Autodesk Inventor part; units mm, degrees
ref_plane "YZ Plane" through (0, 0, 0) normal (1, 0, 0) x (0, 1, 0)
ref_plane "XZ Plane" through (0, 0, 0) normal (0, 1, 0) x (-1, 0, 0)
ref_plane "XY Plane" through (0, 0, 0) normal (0, 0, 1) x (1, 0, 0)
sketch "Sketch1" plane through (0, 0, 0) normal (0, 0, 1) x (1, 0, 0)
  circle A0 centre (0, 0) radius 25
  circle A1 centre (0, 0) radius 35
  line L0 (-17.6777, 17.6777) -> (-24.7487, 24.7487)
  line L1 (0, 35) -> (0, 0) construction
  line L2 (-24.0315, 25.4457) -> (-16.9564, 18.3706)
  line L3 (-1.1667, 34.9806) -> (-1.1667, 34.9972)
  line L4 (1.1667, 34.9806) -> (1.1667, 34.9972)
  line L5 (17.6777, 17.6777) -> (24.7487, 24.7487)
  line L6 (24.0315, 25.4457) -> (16.9564, 18.3706)
  line L7 (-25.4457, 24.0315) -> (-18.3706, 16.9564)
  line L8 (25.4457, 24.0315) -> (18.3706, 16.9564)
  line L9 (-1, 15) -> (1, 15)
  line L10 (1, 15) -> (1, 0)
  line L11 (1, 0) -> (-1, 0)
  line L12 (-1, 0) -> (-1, 15)
  line L13 (-1, 0) -> (1, 0)
  line L14 (1, 0) -> (1, -6)
  line L15 (1, -6) -> (-1, -6)
  line L16 (-1, -6) -> (-1, 0)
  line L17 (-1, -6) -> (-5, -6)
  line L18 (-5, -6) -> (-5, 3)
  line L19 (-5, 3) -> (-1, 3)
  line L20 (-1, 3) -> (-1, -6)
  line L21 (-5, 3) -> (-21.2192, -13.2192)
  line L22 (-5, -6) -> (-17.1706, -18.1706)
  line L23 (-5, 3) -> (-1, 15)
  line L24 (-5, -6) -> (-1, -2)
  line L25 (1, 0) -> (1, 15)
  line L26 (1, -6) -> (1, 0)
  line L27 (5, 3) -> (21.2192, -13.2192)
  line L28 (5, -6) -> (17.1706, -18.1706)
  line L29 (5, 3) -> (1, 15)
  line L30 (5, -6) -> (1, -2)
  point P0 (-20.5061, 21.9203)
  point P1 (-21.9203, 20.5061)
  point P2 (20.5061, 21.9203)
  point P3 (21.9203, 20.5061)
  point P4 (-1, -2)
  point P5 (1, 0)
  point P6 (1, -2)
  dimension "d0" = 50
  dimension "d1" = 10
  dimension "d2" = 45
  dimension "d3" = 1
  dimension "d5" = 2
  dimension "d6" = 15
  dimension "d7" = 6
  dimension "d8" = 2
  dimension "d9" = 4
  dimension "d11" = 45
  dimension "d12" = 45
  dimension "d13" = 3
  dimension "d14" = 45
extrude "Extrusion1" add sketch "Sketch1" along normal blind 5 contours A0 L0 A1 L2 | A1 L0 A0 L7
sketch "Sketch3" plane through (-24.0315, 25.4457, 0) normal (0.7071, 0.7071, 0) x (-0.7071, 0.7071, 0)
  line L0 (-10.0057, 5) -> (0, 5) construction
  line L1 (-10.0057, 0) -> (-10.0057, 5) construction
  circle A0 centre (-5.0029, 2.5) radius 1.4
  point P0 (-34.9857, 0)
  dimension "d19" = 2.8
  dimension "d20" = 2.5
  dimension "d21" = 5.0029
extrude "Extrusion3" add sketch "Sketch3" along normal blind 4.8
chamfer "Chamfer1" distance 1 angle 45 1 edges at (-16.1099, 24.3123, 2.5)
properties part number "Black_Part1"
Geometry check sheet. Reference: the model listing, model coordinates, mm. Give positions to 0.01 mm unless a question says otherwise; leave off trailing zeros. Write each loop counter-clockwise with the first axis right and the second up, starting at its lowest first coordinate (ties: lowest second). Pieces come first, ordered by that corner, then holes.
1) Cross-section at B-B (x = -23.25). Record the boundary of the cut face in (y, z), plus the area to 3 significant figures.
Values follow:
outline: (21.84, 0) - (24.66, 0) - (24.66, 5) - (21.84, 5) - close
area: 14.1 mm2
2) Release check for a two-part mould opening along X. For faces 1 (the face through (-20.1, 24.2, 2.1)), 2 (the face through (-24.8, 24.7, 2.5)), 3 (the face through (-21, 21, 0)), 4 (the face through (-21.33, 22.744, 1.354)) record: released by +X, released by -X, zero draft, split by the parting line, or undercut.
Values follow:
face 1: undercut
face 2: released by -X
face 3: zero draft
face 4: undercut
3) Cross-section at A-A (y = 18.25). Record the boundary of the cut face in (x, z), plus the area to 3 significant figures.
Values follow:
outline: (-19.66, 0) - (-17.09, 0) - (-17.09, 5) - (-19.66, 5) - close
area: 12.9 mm2
4) Thickness scan on line 1 (X direction, y = 23.25, z = 1.95); line 2 (X direction, y = 23.25, z = 1.4); line 3 (Y direction, x = -17.75, z = 3). Record the ranges inside material, lowest first.
Values follow:
line 1: x = -24.66 to -21.84, -20.97 to -17.33
line 2: x = -24.66 to -21.84, -20.38 to -17.93
line 3: y = 17.61 to 19.16, 22.8 to 25.45
